Read the model definition and answer for the solid it produces. Units are mm, in the model's axes. Face numbers are marked on the shaded views. A direction names the side the tool comes from. Coordinates: 2 decimals unless noted, no trailing zeros. Write each loop counter-clockwise with the first axis right and the second up, starting at its lowest first coordinate (ties: lowest second). Pieces come first, ordered by that corner, then holes.
Item 1: A tool of negligible diameter and unlimited length cuts with its end or side. For the marked faces 1, 2, 3, 4 and 5, from which of +Z, -Z, +X, -X, +Y, -Y can it reach the whole face along a straight path? Write none if from no direction.
Item 2: Each of these flat-tipped pins is pushed along its axis until it touches: P1, Ø2, axis at x = -31, y = 2.5, coming from the -Z side; P2, Ø2.5, axis at x = 1.5, y = 12, coming from the -Z side; P3, Ø4, axis at x = 22.5, y = 10.5, coming from the -Z side; P4, Ø7, axis at x = 0, z = -23.32, coming from the +Y side. Where does it stop, or does it pass through?
Item 3: Section D-D (z = 36.5) is taken. Give the vertices of the cut face in (x, y), then the cut area to 3 significant figures.
Item 4: Section C-C (x = 0) is taken. Give the vertices of the cut face in (y, z).
Item 5: Section A-A (x = 31) is taken. Give the vertices of the cut face in (y, z), then the cut area to 3 significant figures.
Item 6: Straight lines are drawn through the part: probe 1 along Z at (x, y) = (0, 4.9); probe 2 along Y at (x, z) = (31, 35); probe 3 along Y at (x, z) = (2, -20). For each, find the intervals that lie inside material, in ascending order.
Item 7: Section B-B (y = 13.5) is taken. Give the vertices of the cut face in (x, z).
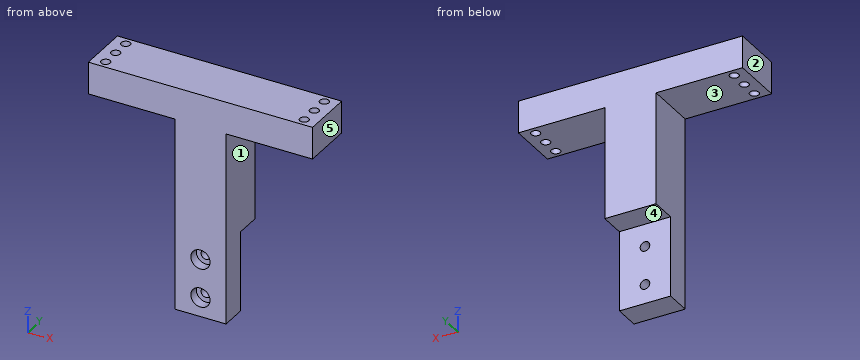
Autodesk Inventor part; units mm, degrees
ref_plane "YZ Plane" through (0, 0, 0) normal (1, 0, 0) x (0, 1, 0)
ref_plane "XZ Plane" through (0, 0, 0) normal (0, 1, 0) x (-1, 0, 0)
ref_plane "XY Plane" through (0, 0, 0) normal (0, 0, 1) x (1, 0, 0)
sketch "Sketch1" plane through (0, 0, 0) normal (0, 1, 0) x (-1, 0, 0)
  line L0 (0, -29.3233) -> (8, -29.3233)
  line L1 (8, -29.3233) -> (8, 30.6767)
  line L2 (0, 0) -> (0, -29.3233) construction
  line L3 (0, -29.3233) -> (-8, -29.3233)
  line L4 (-8, -29.3233) -> (-8, 30.6767)
  line L5 (8, 30.6767) -> (35, 30.6767)
  line L6 (35, 30.6767) -> (35, 40.6767)
  line L7 (35, 40.6767) -> (2.1646, 40.6767)
  line L8 (2.1646, 40.6767) -> (0, 40.6767)
  line L9 (-8, 30.6767) -> (-35, 30.6767)
  line L10 (-35, 30.6767) -> (-35, 40.6767)
  line L11 (-35, 40.6767) -> (-2.1646, 40.6767)
  line L12 (-2.1646, 40.6767) -> (0, 40.6767)
  point P0 (4, -29.3233)
  point P1 (-4, -29.3233)
  dimension "d0" = 16
  dimension "d17" = 10
  dimension "d32" = 70
  dimension "d35" = 70
extrude "Extrusion1" add sketch "Sketch1" along normal blind 16
sketch "Sketch2" plane through (0, 16, 0) normal (0, 1, 0) x (1, 0, 0)
  line L0 (8, 29.3233) -> (-8, 29.3233)
  line L1 (-8, 29.3233) -> (-8, -30.6767)
  line L2 (8, -30.6767) -> (8, 29.3233)
  line L3 (8, -30.6767) -> (8, 29.3233)
  line L4 (-8, 29.3233) -> (8, 29.3233)
  line L5 (8, 29.3233) -> (8, 4.3233)
  line L6 (8, 4.3233) -> (-8, 4.3233)
  line L7 (-8, 4.3233) -> (-8, 29.3233)
  line L8 (-8, -30.6767) -> (-35, -30.6767)
  line L9 (-35, -30.6767) -> (-35, -40.6767)
  line L10 (-35, -40.6767) -> (35, -40.6767)
  line L11 (35, -40.6767) -> (35, -30.6767)
  line L12 (35, -30.6767) -> (8, -30.6767)
  point P0 (0, 0)
  point P1 (-8, 4.3233)
  dimension "d6" = 25
extrude "Extrusion2" cut sketch "Sketch2" against normal blind 8 contours L2 L6 L1 L0
sketch "Sketch3" plane through (0, 0, 0) normal (0, -1, 0) x (1, 0, 0)
  line L0 (8, -29.3233) -> (-8, -29.3233)
  line L1 (8, 30.6767) -> (8, -29.3233)
  line L2 (-8, -29.3233) -> (-8, 30.6767)
  circle A0 centre (0, -23.3233) radius 1.5
  circle A1 centre (0, -11.3233) radius 1.5
  line L3 (35, 30.6767) -> (8, 30.6767)
  line L4 (35, 40.6767) -> (35, 30.6767)
  line L5 (-35, 40.6767) -> (35, 40.6767)
  line L6 (-35, 30.6767) -> (-35, 40.6767)
  line L7 (-8, 30.6767) -> (-35, 30.6767)
  point P0 (0, 0)
  dimension "d9" = 3
  dimension "d10" = 6
  dimension "d11" = 12
extrude "Extrusion3" cut sketch "Sketch3" against normal through all contours A0 | A1
sketch "Sketch4" plane through (0, 0, 0) normal (0, -1, 0) x (1, 0, 0)
  circle A0 centre (0, -11.3233) radius 1.5
  circle A1 centre (0, -23.3233) radius 1.5
  line L0 (8, -29.3233) -> (-8, -29.3233)
  line L1 (8, 30.6767) -> (8, -29.3233)
  line L2 (-8, -29.3233) -> (-8, 30.6767)
  circle A2 centre (0, -23.3233) radius 3
  circle A3 centre (0, -11.3233) radius 1.5
  circle A4 centre (0, -11.3233) radius 3
  line L3 (35, 30.6767) -> (8, 30.6767)
  line L4 (35, 40.6767) -> (35, 30.6767)
  line L5 (-35, 40.6767) -> (35, 40.6767)
  line L6 (-35, 30.6767) -> (-35, 40.6767)
  line L7 (-8, 30.6767) -> (-35, 30.6767)
  point P0 (0, 0)
  dimension "d14" = 6
extrude "Extrusion4" cut sketch "Sketch4" against normal blind 3 contours A2 | A4
sketch "Sketch5" plane through (0.8354, 0, 40.6767) normal (0, 0, 1) x (1, 0, 0)
  line L0 (-35.8354, 0) -> (34.1646, 0)
  line L1 (-35.8354, 16) -> (34.1646, 16)
  line L2 (-35.8354, 0) -> (-35.8354, 16)
  line L3 (-35.8354, 0) -> (-35.8354, 16) construction
  line L4 (-35.8354, 8) -> (34.1646, 8) construction
  circle A0 centre (-31.8354, 13.5) radius 1.4
  circle A1 centre (-31.8354, 8) radius 1.4
  circle A2 centre (-31.8354, 2.5) radius 1.4
  line L5 (34.1646, 0) -> (34.1646, 16)
  line L6 (-35.8354, 16) -> (34.1646, 16) construction
  line L7 (-0.8354, 16) -> (-0.8354, 0) construction
  line L8 (-35.8354, 0) -> (34.1646, 0)
  circle A3 centre (30.1646, 13.5) radius 1.4
  circle A4 centre (30.1646, 8) radius 1.4
  circle A5 centre (30.1646, 2.5) radius 1.4
  dimension "d19" = 2.8
  dimension "d20" = 11
  dimension "d21" = 4
extrude "Extrusion8" cut sketch "Sketch5" against normal through all contours A0 | A1 | A2 | A3 | A4 | A5
properties part number "B1_head_T"
Established:
1. face 1: -Z, +X, +Y, -Y
1. face 2: +Z, -Z, -X, +Y, -Y
1. face 3: -Z, -X, +Y, -Y
1. face 4: -Z, +X, -X, +Y
1. face 5: +Z, -Z, +X, +Y, -Y
2. P1: passes through
2. P2: stops at z = -4.32
2. P3: stops at z = 30.68
2. P4: stops at y = 8
3. outline: (-35, 0) - (35, 0) - (35, 16) - (-35, 16) - close; hole circle Ø2.8 at (-31, 2.5); hole circle Ø2.8 at (-31, 8); hole circle Ø2.8 at (-31, 13.5); hole circle Ø2.8 at (31, 2.5); hole circle Ø2.8 at (31, 8); hole circle Ø2.8 at (31, 13.5)
3. area: 1,080 mm2
4. outline: (0, -29.32) - (8, -29.32) - (8, -24.82) - (3, -24.82) - (3, -26.32) - (0, -26.32) - close; (0, -20.32) - (3, -20.32) - (3, -21.82) - (8, -21.82) - (8, -12.82) - (3, -12.82) - (3, -14.32) - (0, -14.32) - close; (0, -8.32) - (3, -8.32) - (3, -9.82) - (8, -9.82) - (8, -4.32) - (16, -4.32) - (16, 40.68) - (0, 40.68) - close
5. outline: (0, 30.68) - (1.1, 30.68) - (1.1, 40.68) - (0, 40.68) - close; (3.9, 30.68) - (6.6, 30.68) - (6.6, 40.68) - (3.9, 40.68) - close; (9.4, 30.68) - (12.1, 30.68) - (12.1, 40.68) - (9.4, 40.68) - close; (14.9, 30.68) - (16, 30.68) - (16, 40.68) - (14.9, 40.68) - close
5. area: 76.0 mm2
6. probe 1: z = -29.32 to -24.82, -21.82 to -12.82, -9.82 to 40.68
6. probe 2: y = 0 to 1.1, 3.9 to 6.6, 9.4 to 12.1, 14.9 to 16
6. probe 3: y = 0 to 8
7. outline: (-35, 30.68) - (-32.4, 30.68) - (-32.4, 40.68) - (-35, 40.68) - close; (-29.6, 30.68) - (-8, 30.68) - (-8, -4.32) - (8, -4.32) - (8, 30.68) - (29.6, 30.68) - (29.6, 40.68) - (-29.6, 40.68) - close; (32.4, 30.68) - (35, 30.68) - (35, 40.68) - (32.4, 40.68) - close
